Can you work these out from the drawing? Everything is in mm from the part's minimum corner. A direction names the side the tool comes from. Coordinates: 2 decimals unless noted, no trailing zeros. Loops run counter-clockwise (first coordinate to the right, second up) from the corner with the lowest first, then second, coordinate; pieces in that order, holes last. Notation, with made-up numbers: (33, 87) - (79, 87) arc R20 ccw to (79, 119) - close; hole circle Ø3 at (76, 42.25). An arc over 180 degrees is marked (long way). Put each result on its own line as item: value. Start each with the question number.
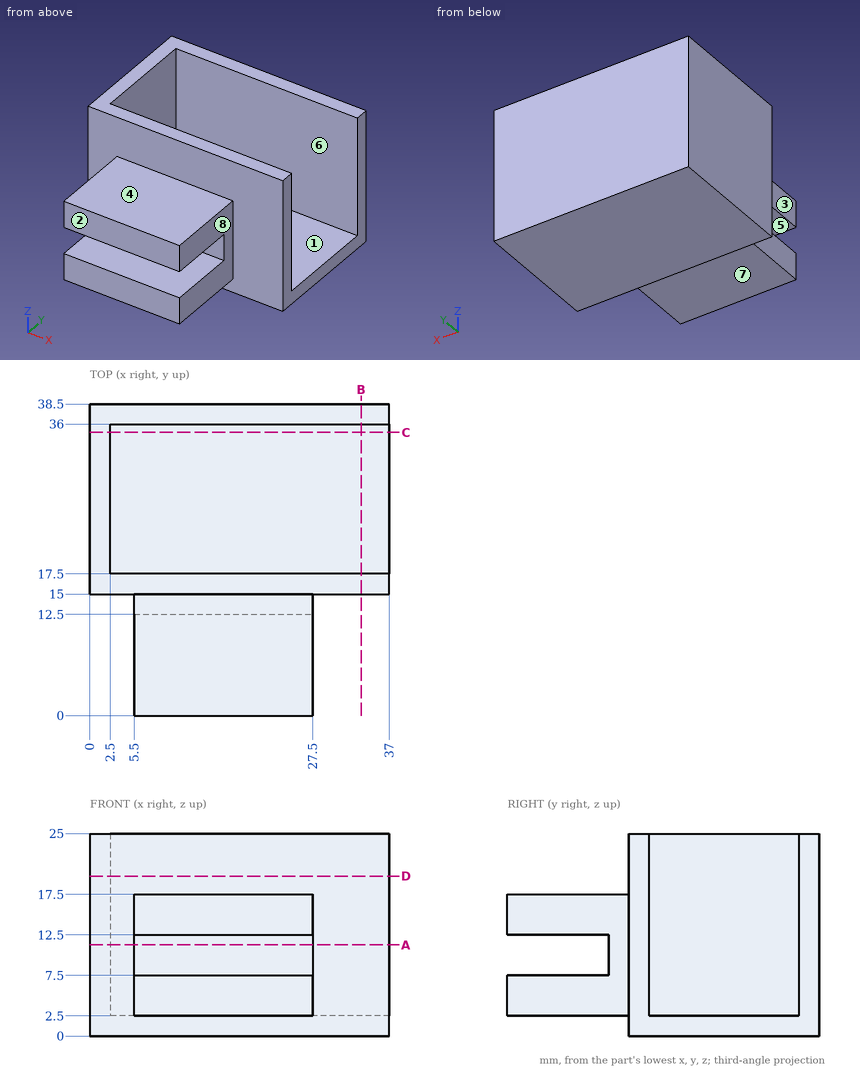
Q1. Will these pins go through, and if not, where does the flat tip stop? pin 1 (12 mm diameter, centred on x = 19, y = 4, fed in from +Z); pin 2 (1 mm diameter, centred on y = 32, z = 13, fed in from +X); pin 3 (5 mm diameter, centred on x = 28, z = 21.5, fed in from -Y); pin 4 (1.5 mm diameter, centred on y = 7, z = 10, fed in from -X).
Q2. We'd pull the mould along Y, two halves only. Please class the marked faces 1, 2 and 3: released by +Y, released by -Y, zero draft, split by the parting line, or undercut.
Q3. I want a section at B-B on x = 33.5. List the corners of the cut face in (y, z) for me, and give its area (3 significant figures).
Q4. Please list where these lines run through material, in increasing order: line 1 along Y through (x, z) = (33.5, 23.5); line 2 along Z through (x, y) = (22, 2); line 3 along Y through (x, z) = (21.5, 12.25). Write a range as [from, to].
Q5. I want a section at D-D on z = 19.75. List the corners of the cut face in (x, y) for me.
Q6. On a 3-axis mill with a long thin cutter (end or side, diameter ignored), from which of +Z, -Z, +X, -X, +Y, -Y can I reach the whole of each face in a straight line? I mean the marked faces 4, 5, 6, 7 and 8. Say none if no direction works.
Q7. I want a section at A-A on z = 11.25. List the corners of the cut face in (x, y) for me, and give its area (3 significant figures).
Q8. I want a section at C-C on y = 35. List the corners of the cut face in (x, z) for me.
Calculated:
1. pin 1: z = 17.5
1. pin 2: x = 2.5
1. pin 3: y = 15
1. pin 4: through
2. face 1: undercut
2. face 2: released by -Y
2. face 3: zero draft
3. outline: (15, 0) - (38.5, 0) - (38.5, 25) - (36, 25) - (36, 2.5) - (17.5, 2.5) - (17.5, 25) - (15, 25) - close
3. area: 171 mm2
4. line 1: [15, 17.5], [36, 38.5]
4. line 2: [2.5, 7.5], [12.5, 17.5]
4. line 3: [12.5, 17.5], [36, 38.5]
5. outline: (0, 15) - (37, 15) - (37, 17.5) - (2.5, 17.5) - (2.5, 36) - (37, 36) - (37, 38.5) - (0, 38.5) - close
6. face 4: +Z, +X, -X, -Y
6. face 5: +X, -X, -Y
6. face 6: +Z, +X
6. face 7: -Z, +X, -X, -Y
6. face 8: +Z, -Z, +X, -Y
7. outline: (0, 15) - (5.5, 15) - (5.5, 12.5) - (27.5, 12.5) - (27.5, 15) - (37, 15) - (37, 17.5) - (2.5, 17.5) - (2.5, 36) - (37, 36) - (37, 38.5) - (0, 38.5) - close
7. area: 286 mm2
8. outline: (0, 0) - (37, 0) - (37, 2.5) - (2.5, 2.5) - (2.5, 25) - (0, 25) - close
